```python
from build123d import *

# Parameters (mm, degrees)
SKETCH1_R           = 15.584715873
SKETCH1_R_2         = 1.25
SKETCH1_R_3         = 33.3375
SKETCH1_R_4         = 2.25
SKETCH1_R_5         = 1.65
SKETCH1_R_6         = 20.6375
BOSS_EXTRUDE1_DEPTH = 6.35
BOSS_EXTRUDE2_START = -6.35
SKETCH1_3_R         = 33.3375
SKETCH1_3_R_2       = 2.25
SKETCH1_3_R_3       = 1.65
SKETCH1_3_R_4       = 20.6375
SKETCH1_3_R_5       = 15.584715873
SKETCH1_3_R_6       = 1.25
BOSS_EXTRUDE2_DEPTH = 6.35


with BuildPart() as part:
    # Sketch1 → Boss-Extrude1 (new body)
    # profile 1 of 3: a face of its own
    with BuildSketch(Plane.XY):
        with Locations((-76.366650528, -0.386154045)):
            Circle(SKETCH1_R)
        with Locations((-67.489890139, 4.738845955)):
            Circle(SKETCH1_R_2, mode=Mode.SUBTRACT)
        with Locations((-67.489890139, -5.511154045)):
            Circle(SKETCH1_R_2, mode=Mode.SUBTRACT)
        with Locations((-76.366650528, -10.636154045)):
            Circle(SKETCH1_R_2, mode=Mode.SUBTRACT)
        with Locations((-85.243410916, -5.511154045)):
            Circle(SKETCH1_R_2, mode=Mode.SUBTRACT)
        with Locations((-85.243410916, 4.738845955)):
            Circle(SKETCH1_R_2, mode=Mode.SUBTRACT)
        with Locations((-76.366650528, 9.863845955)):
            Circle(SKETCH1_R_2, mode=Mode.SUBTRACT)
        Polygon((-79.366650528, -2.118204852), (-79.366650528, 1.345896763), (-76.366650528, 3.07794757), (-73.366650528, 1.345896763), (-73.366650528, -2.118204852), (-76.366650528, -3.85025566), align=None, mode=Mode.SUBTRACT)
    # profile 2 of 3: a face of its own
    with BuildSketch(Plane.XY):
        with BuildLine():
            Line((21.162931467, 15.198561829), (-76.366650528, 15.198561829))
            ThreePointArc((-76.366650528, 15.198561829), (-65.346592251, 10.633904232), (-60.781934654, -0.386154045))
            ThreePointArc((-60.781934654, -0.386154045), (-65.346592251, -11.406212322), (-76.366650528, -15.970869918))
            Line((-76.366650528, -15.970869918), (21.162931467, -15.970869918))
            ThreePointArc((21.162931467, -15.970869918), (17.295849472, -0.386154045), (21.162931467, 15.198561829))
        make_face()
        with BuildLine():
            ThreePointArc((-50.966650528, -4.831154045), (-55.411650528, -0.386154045), (-50.966650528, 4.058845955))
            Line((-50.966650528, 4.058845955), (6.183349472, 4.058845955))
            ThreePointArc((6.183349472, 4.058845955), (10.628349472, -0.386154045), (6.183349472, -4.831154045))
            Line((6.183349472, -4.831154045), (-50.966650528, -4.831154045))
        make_face(mode=Mode.SUBTRACT)
    # profile 3 of 3: a face of its own
    with BuildSketch(Plane.XY):
        with Locations((50.633349472, -0.386154045)):
            Circle(SKETCH1_R_3)
        with Locations((32.955679943, 17.291515485)):
            Circle(SKETCH1_R_4, mode=Mode.SUBTRACT)
        with Locations((68.311019002, 17.291515485)):
            Circle(SKETCH1_R_5, mode=Mode.SUBTRACT)
        with Locations((68.311019002, -18.063823575)):
            Circle(SKETCH1_R_4, mode=Mode.SUBTRACT)
        with Locations((32.955679943, -18.063823575)):
            Circle(SKETCH1_R_5, mode=Mode.SUBTRACT)
        with Locations((50.633349472, -0.386154045)):
            Circle(SKETCH1_R_6, mode=Mode.SUBTRACT)
    extrude(amount=BOSS_EXTRUDE1_DEPTH)

    # Sketch1_3 → Boss-Extrude2 (add)
    # profile 1 of 2: a face of its own
    with BuildSketch(Plane.XY.offset(BOSS_EXTRUDE2_START)):
        with Locations(Location((50.633349472, -0.386154045, 0), (0, 0, 207.871038918))):
            Circle(SKETCH1_3_R)
        with Locations((32.955679943, 17.291515485)):
            Circle(SKETCH1_3_R_2, mode=Mode.SUBTRACT)
        with Locations((68.311019002, 17.291515485)):
            Circle(SKETCH1_3_R_3, mode=Mode.SUBTRACT)
        with Locations((68.311019002, -18.063823575)):
            Circle(SKETCH1_3_R_2, mode=Mode.SUBTRACT)
        with Locations((32.955679943, -18.063823575)):
            Circle(SKETCH1_3_R_3, mode=Mode.SUBTRACT)
        with Locations((50.633349472, -0.386154045)):
            Circle(SKETCH1_3_R_4, mode=Mode.SUBTRACT)
    # profile 2 of 2: a face of its own
    with BuildSketch(Plane.XY.offset(BOSS_EXTRUDE2_START)):
        with Locations(Location((-76.366650528, -0.386154045, 0), (0, 0, 90))):
            Circle(SKETCH1_3_R_5)
        with Locations((-67.489890139, 4.738845955)):
            Circle(SKETCH1_3_R_6, mode=Mode.SUBTRACT)
        with Locations((-67.489890139, -5.511154045)):
            Circle(SKETCH1_3_R_6, mode=Mode.SUBTRACT)
        with Locations((-76.366650528, -10.636154045)):
            Circle(SKETCH1_3_R_6, mode=Mode.SUBTRACT)
        with Locations((-85.243410916, -5.511154045)):
            Circle(SKETCH1_3_R_6, mode=Mode.SUBTRACT)
        with Locations((-85.243410916, 4.738845955)):
            Circle(SKETCH1_3_R_6, mode=Mode.SUBTRACT)
        with Locations((-76.366650528, 9.863845955)):
            Circle(SKETCH1_3_R_6, mode=Mode.SUBTRACT)
        Polygon((-79.366650528, -2.118204852), (-79.366650528, 1.345896763), (-76.366650528, 3.07794757), (-73.366650528, 1.345896763), (-73.366650528, -2.118204852), (-76.366650528, -3.85025566), align=None, mode=Mode.SUBTRACT)
    extrude(amount=BOSS_EXTRUDE2_DEPTH)


solid = part.part
```
Design review of the part built by this model. Coordinates are the model's own, in mm. A direction names the side the tool comes from. Give positions to 0.01 mm unless a question says otherwise; leave off trailing zeros. Order: outer loops, then holes, each group sorted by start corner. A loop starts at its lowest first (then second) coordinate and runs counter-clockwise, first axis right, second up. Notation, with made-up numbers: (40.25, 23.5) -> (94.25, 23.5) arc R18 ccw to (94.25, 41.5) -> close; hole circle Ø9 at (57, -17.5). An arc over 180 degrees is marked (long way). Write each question's results on one line, items separated by ' | '. Start each with the question number.
Q1. Add section A-A on z = -3.25. State how many separate pieces and enclosed holes the cut face has, and give its area (3 significant figures).
Q2. Add section D-D on x = 46.5. Give the boundary of the cut face in (y, z).
Q3. Machinability: for faces 5 (the flat face through (-73, -1, -6.35)), 6 (the flat face through (-27, 15.199, 3)), 7 (the cylindrical face through (-91.82, -2.41, -1.5)), 8 (the flat face through (-23, 4.059, 3)), which of the approach directions +Z, -Z, +X, -X, +Y, -Y give a long, thin tool a straight path to every point of the face, cutting with its end or side? Answer none if there is none.
Q4. Wall thickness on L1, parallel to X at y = -1, z = -2.5; L2, parallel to X at y = -3, z = 5.5; L3, parallel to Y at x = -7, z = 5: over which ranges is each line inside the solid? List them lowest first. Write a range as from..to.
Q5. Add section C-C on y = 13. Give the boundary of the cut face in (x, z), and give its area (3 significant figures).
Q6. For pin 1 (1.9 mm diameter, centred on x = -15.5, z = 4, fed in from -Y); pin 2 (7 mm diameter, centred on x = -49, z = 3, fed in from +Y); pin 3 (3 mm diameter, centred on x = 9.5, y = 11, fed in from -Z), all flat-tipped, find the tip position at first contact; note any pin that passes through.
Q7. Add section B-B on x = -17. Give the boundary of the cut face in (y, z), and give its area (3 significant figures).
Q8. Mouldability with a two-part tool opening along Y and no side actions: class faces 1 (the flat face through (-28, -15.971, 3)), 2 (the cylindrical face through (66.5, -19.4, -0.1)), 3 (the flat face through (45, -21, -6.35)), 4 (the cylindrical face through (31.17, 15.92, -0.09)) as +Y half, -Y half, draft (parallel to the pull), parting line (faces both ways), or undercut.
Found:
1) separate pieces: 2 | enclosed holes: 12 | area: 2,810 mm2
2) outline: (-33.47, -6.35) -> (-20.61, -6.35) -> (-20.61, 6.35) -> (-33.47, 6.35) -> close; (19.83, -6.35) -> (32.69, -6.35) -> (32.69, 6.35) -> (19.83, 6.35) -> close
3) face 5: -Z, +X, -X, +Y, -Y | face 6: +Z, -Z, -X, +Y | face 7: -Z | face 8: +Z, -Z
4) L1: x = -91.94..-79.37, -73.37..-60.79, 17.3..30, 71.26..83.97 | L2: x = -91.73..-77.84, -74.89..-54.56, 9.78..30.16, 71.1..83.87 | L3: y = -15.97..-4.83, 4.06..15.2
5) outline: (-84.35, -6.35) -> (-68.39, -6.35) -> (-68.39, 0) -> (20.1, 0) -> (20.1, -6.35) -> (34.93, -6.35) -> (34.93, 6.35) -> (-84.35, 6.35) -> close; (66.34, -6.35) -> (81.17, -6.35) -> (81.17, 6.35) -> (66.34, 6.35) -> close | area: 1,140 mm2
6) pin 1: stops at y = -15.97 | pin 2: stops at y = 15.2 | pin 3: stops at z = 0
7) outline: (-15.97, 0) -> (-4.83, 0) -> (-4.83, 6.35) -> (-15.97, 6.35) -> close; (4.06, 0) -> (15.2, 0) -> (15.2, 6.35) -> (4.06, 6.35) -> close | area: 141 mm2
8) face 1: -Y half | face 2: undercut | face 3: draft | face 4: undercut
